```python
from build123d import *

# Parameters (mm, degrees)
F1_DEPTH  = 1.2
F2_DEPTH  = 9
F4_DEPTH  = 1.2
F5_W      = 10
F5_H      = 5
F6_DEPTH  = 1.2
F7_W      = 9
F7_H      = 1
F8_DEPTH  = 1.2
F9_W      = 15
F9_H      = 8
F10_DEPTH = 1.2
F11_R     = 3
F12_DEPTH = 1.2
F14_DEPTH = 9.001


with BuildPart() as f1:
    # F0 (on Top) → F1 (new body)
    with BuildSketch(Plane.XY):
        with BuildLine():
            Line((-31.6, -72.8), (31.6, -72.8))
            ThreePointArc((31.6, -72.8), (35.1355339059, -71.3355339059), (36.6, -67.8))
            Line((36.6, -67.8), (36.6, 67.8))
            ThreePointArc((36.6, 67.8), (35.1355339059, 71.3355339059), (31.6, 72.8))
            Line((31.6, 72.8), (-31.6, 72.8))
            ThreePointArc((-31.6, 72.8), (-35.1355339059, 71.3355339059), (-36.6, 67.8))
            Line((-36.6, 67.8), (-36.6, -67.8))
            ThreePointArc((-36.6, -67.8), (-35.1355339059, -71.3355339059), (-31.6, -72.8))
        make_face()
        with BuildLine():
            ThreePointArc((35.4, -66.6), (33.9355339059, -70.1355339059), (30.4, -71.6))
            Line((30.4, -71.6), (-30.4, -71.6))
            ThreePointArc((-30.4, -71.6), (-33.9355339059, -70.1355339059), (-35.4, -66.6))
            Line((-35.4, -66.6), (-35.4, 66.6))
            ThreePointArc((-35.4, 66.6), (-33.9355339059, 70.1355339059), (-30.4, 71.6))
            Line((-30.4, 71.6), (30.4, 71.6))
            ThreePointArc((30.4, 71.6), (33.9355339059, 70.1355339059), (35.4, 66.6))
            Line((35.4, 66.6), (35.4, -66.6))
        make_face(mode=Mode.SUBTRACT)
        with BuildLine():
            Line((-30.4, -71.6), (30.4, -71.6))
            ThreePointArc((30.4, -71.6), (33.9355339059, -70.1355339059), (35.4, -66.6))
            Line((35.4, -66.6), (35.4, 66.6))
            ThreePointArc((35.4, 66.6), (33.9355339059, 70.1355339059), (30.4, 71.6))
            Line((30.4, 71.6), (-30.4, 71.6))
            ThreePointArc((-30.4, 71.6), (-33.9355339059, 70.1355339059), (-35.4, 66.6))
            Line((-35.4, 66.6), (-35.4, -66.6))
            ThreePointArc((-35.4, -66.6), (-33.9355339059, -70.1355339059), (-30.4, -71.6))
        make_face()
    extrude(amount=F1_DEPTH)

    # F0 (on Top) → F2 (join)
    with BuildSketch(Plane.XY):
        with BuildLine():
            Line((-31.6, -72.8), (31.6, -72.8))
            ThreePointArc((31.6, -72.8), (35.1355339059, -71.3355339059), (36.6, -67.8))
            Line((36.6, -67.8), (36.6, 67.8))
            ThreePointArc((36.6, 67.8), (35.1355339059, 71.3355339059), (31.6, 72.8))
            Line((31.6, 72.8), (-31.6, 72.8))
            ThreePointArc((-31.6, 72.8), (-35.1355339059, 71.3355339059), (-36.6, 67.8))
            Line((-36.6, 67.8), (-36.6, -67.8))
            ThreePointArc((-36.6, -67.8), (-35.1355339059, -71.3355339059), (-31.6, -72.8))
        make_face()
        with BuildLine():
            ThreePointArc((35.4, -66.6), (33.9355339059, -70.1355339059), (30.4, -71.6))
            Line((30.4, -71.6), (-30.4, -71.6))
            ThreePointArc((-30.4, -71.6), (-33.9355339059, -70.1355339059), (-35.4, -66.6))
            Line((-35.4, -66.6), (-35.4, 66.6))
            ThreePointArc((-35.4, 66.6), (-33.9355339059, 70.1355339059), (-30.4, 71.6))
            Line((-30.4, 71.6), (30.4, 71.6))
            ThreePointArc((30.4, 71.6), (33.9355339059, 70.1355339059), (35.4, 66.6))
            Line((35.4, 66.6), (35.4, -66.6))
        make_face(mode=Mode.SUBTRACT)
    extrude(amount=F2_DEPTH)

    # F3 (on face) → F4 (cut, through all)
    with BuildSketch(Plane.YZ.offset(36.6)):
        Polygon((19.8, 2), (26.1, 2), (45.8, 2), (45.8, 7), (26.1, 7), (19.8, 7), (10.8, 7), (10.8, 2), align=None)
    extrude(amount=-F4_DEPTH, mode=Mode.SUBTRACT)

    # F5 (on face) → F6 (cut, through all)
    with BuildSketch(Plane.XZ.offset(72.8)):
        with Locations((0, 4.5)):
            Rectangle(F5_W, F5_H)
    extrude(amount=-F6_DEPTH, mode=Mode.SUBTRACT)

    # F7 (on face) → F8 (cut, through all)
    with BuildSketch(Plane.XZ.offset(72.8)):
        with Locations((-17, 4.5)):
            Rectangle(F7_W, F7_H)
        with Locations((17, 4.5)):
            Rectangle(F7_W, F7_H)
    extrude(amount=-F8_DEPTH, mode=Mode.SUBTRACT)

    # F9 (on face) → F10 (cut, through all)
    with BuildSketch(Plane(origin=(0, 0, 0), x_dir=(1, 0, 0), z_dir=(0, 0, -1))):
        with Locations((20.1, -64.8)):
            Rectangle(F9_W, F9_H)
    extrude(amount=-F10_DEPTH, mode=Mode.SUBTRACT)

    # F11 (on face) → F12 (cut, through all)
    with BuildSketch(Plane(origin=(0, 72.8, 0), x_dir=(-1, 0, 0), z_dir=(0, 1, 0))):
        with Locations((12.6, 4.5)):
            Circle(F11_R)
    extrude(amount=-F12_DEPTH, mode=Mode.SUBTRACT)

    # F13 (on face) → F14 (cut, through all)
    with BuildSketch(Plane.XY.offset(9)):
        with BuildLine():
            Line((-36.6, 67.8), (-36.6, -67.8))
            ThreePointArc((-36.6, -67.8), (-35.1355339059, -71.3355339059), (-31.6, -72.8))
            Line((-31.6, -72.8), (31.6, -72.8))
            ThreePointArc((31.6, -72.8), (35.1355339059, -71.3355339059), (36.6, -67.8))
            Line((36.6, -67.8), (36.6, 67.8))
            ThreePointArc((36.6, 67.8), (35.1355339059, 71.3355339059), (31.6, 72.8))
            Line((31.6, 72.8), (-31.6, 72.8))
            ThreePointArc((-31.6, 72.8), (-35.1355339059, 71.3355339059), (-36.6, 67.8))
        make_face()
        with BuildLine():
            Line((-31.6, 72.4), (31.6, 72.4))
            ThreePointArc((31.6, 72.4), (34.8526911935, 71.0526911935), (36.2, 67.8))
            Line((36.2, 67.8), (36.2, -67.8))
            ThreePointArc((36.2, -67.8), (34.8526911935, -71.0526911935), (31.6, -72.4))
            Line((31.6, -72.4), (-31.6, -72.4))
            ThreePointArc((-31.6, -72.4), (-34.8526911935, -71.0526911935), (-36.2, -67.8))
            Line((-36.2, -67.8), (-36.2, 67.8))
            ThreePointArc((-36.2, 67.8), (-34.8526911935, 71.0526911935), (-31.6, 72.4))
        make_face(mode=Mode.SUBTRACT)
    extrude(amount=-F14_DEPTH, mode=Mode.SUBTRACT)


solid = f1.part
```
Check sheet for the modelled part. Datum: model origin and axes. Units: mm. A direction names the side the tool comes from. Round coordinates to 2 decimals unless told otherwise and drop trailing zeros. Order: outer loops, then holes, each group sorted by start corner. A loop starts at its lowest first (then second) coordinate and runs counter-clockwise, first axis right, second up. Notation, with made-up numbers: (67, 78) -> (94, 78) arc R10 cw to (94, 91) -> close; hole circle Ø9 at (12, 72.5). An arc over 180 degrees is marked (long way). One line per item, written item: value. Start each with the question number.
Q1. Set-up check for faces 5 (the face through (0, 71.6, 5)), 6 (the face through (-9.6, 72, 4.6)), 7 (the face through (34.888, -71.017, 4.563)): record each of +Z, -Z, +X, -X, +Y, -Y from which the full face is reachable in a straight line by a thin tool's end or side.
Q2. Cross-section at B-B (y = 42). Record the boundary of the cut face in (x, z), and give its area (3 significant figures).
Q3. Mould release check, pull along X, two halves, no side actions. Record for faces 1 (the face through (0, 72.4, 5)), 2 (the face through (0, -71.6, 8)), 3 (the face through (-36.2, -1, 5)), 4 (the face through (-33.9, -70.17, 5.05)): pulls with the +X half, pulls with the -X half, needs draft (parallel to the pull), parting line crosses it, or undercut.
Q4. Gauge pin test, flat ends, axial feed: pin 1 Ø0.9 at (x, z) = (36, 4.5) entering from -Y; pin 2 Ø8 at (x, y) = (-22, -38.5) entering from +Z; pin 3 Ø0.9 at (y, z) = (-72, 3.5) entering from +X. Record the tip position at first contact, or that the pin passes through.
Q5. Thickness scan on line 1 (X direction, y = 53.5, z = 6); line 2 (Y direction, x = -18, z = 2.5); line 3 (Z direction, x = -12.6, y = 71.95). Record the ranges inside material, lowest first.
Q6. Cross-section at A-A (x = 25). Record the boundary of the cut face in (y, z), and give its area (3 significant figures).
Q7. Cross-section at C-C (y = -34.5). Record the boundary of the cut face in (x, z).
Completed:
1. face 5: +Z
1. face 6: +Y
1. face 7: +Z, -Z, +X, -Y
2. outline: (-36.2, 0) -> (36.2, 0) -> (36.2, 2) -> (35.4, 2) -> (35.4, 1.2) -> (-35.4, 1.2) -> (-35.4, 9) -> (-36.2, 9) -> close; (35.4, 7) -> (36.2, 7) -> (36.2, 9) -> (35.4, 9) -> close
2. area: 95.4 mm²
3. face 1: needs draft
3. face 2: undercut
3. face 3: pulls with the -X half
3. face 4: undercut
4. pin 1: stops at y = -70.16
4. pin 2: stops at z = 1.2
4. pin 3: stops at x = 34.26
5. line 1: x = -36.2 to -35.4, 35.4 to 36.2
5. line 2: y = -72.4 to -71.6, 71.6 to 72.4
5. line 3: z = 0 to 1.5, 7.5 to 9
6. outline: (-72.4, 0) -> (60.8, 0) -> (60.8, 1.2) -> (-71.6, 1.2) -> (-71.6, 9) -> (-72.4, 9) -> close; (68.8, 0) -> (72.4, 0) -> (72.4, 9) -> (71.6, 9) -> (71.6, 1.2) -> (68.8, 1.2) -> close
6. area: 177 mm²
7. outline: (-36.2, 0) -> (36.2, 0) -> (36.2, 9) -> (35.4, 9) -> (35.4, 1.2) -> (-35.4, 1.2) -> (-35.4, 9) -> (-36.2, 9) -> close
